Design review of the part built by this model. Coordinates are the model's own, in mm. A direction names the side the tool comes from. Give positions to 0.01 mm unless a question says otherwise; leave off trailing zeros. Order: outer loops, then holes, each group sorted by start corner. A loop starts at its lowest first (then second) coordinate and runs counter-clockwise, first axis right, second up. Notation, with made-up numbers: (-24.75, 83) -> (-17.75, 83) arc R29 ccw to (-17.75, 119) -> close; hole circle Ø1 at (61.25, -16). An arc over 180 degrees is marked (long way). One line per item, written item: value. Start each with the question number.
1) Tool access review of faces 1 (the face through (3, 4.3, -3)), 2 (the face through (149, 4, 10.3)), 3 (the face through (84, 0, 0)): name each direction out of +Z, -Z, +X, -X, +Y, -Y from which nothing blocks a thin tool from reaching the whole face with its end or side.
2) For pin 1 (3 mm diameter, centred on y = 2, z = 4.5, fed in from +X); pin 2 (1.8 mm diameter, centred on x = -6, z = 5.5, fed in from +Y); pin 3 (2 mm diameter, centred on x = 173.25, z = 5, fed in from +Y), all flat-tipped, find the tip position at first contact; note any pin that passes through.
3) The part is to be moulded in two halves that separate along Z. For faces 4 (the face through (-10.74, 6.18, -2.38)), 5 (the face through (84, 4, 17)), 6 (the face through (84, 8, 0)), say which applies: released by +Z, released by -Z, zero draft, split by the parting line, or undercut.
4) Consider section A-A (z = 0). State the section outline as (x, y) points.
5) Wall thickness on line 1 along Z through (x, y) = (125.75, 3.75); line 2 along Z through (x, y) = (153, 5); line 3 along X through (y, z) = (3, -5): over which ranges is each line inside the solid? List them lowest first. Write a range as from..to.
6) Consider section D-D (x = 173.25). State the section outline as (y, z) points, plus the area to 3 significant figures.
7) Consider section C-C (x = 139). State the section outline as (y, z) points, plus the area to 3 significant figures.
8) Consider section B-B (y = 2.5). State how many separate pieces and enclosed holes the cut face has, plus the area to 3 significant figures.
from build123d import *

# Parameters (mm, degrees)
ESTRUSIONE_ESTRUSIONE1_DEPTH  = 8
TAGLIO_ESTRUSIONE1_DEPTH      = 183.967210177
TAGLIO_ESTRUSIONE1_DEPTH_BACK = 183.967210177
SCHIZZO2_R                    = 3.5
SCHIZZO2_W                    = 41.6
SCHIZZO2_H                    = 20.6
SCHIZZO3_R                    = 11
TAGLIO_ESTRUSIONE2_DEPTH      = 3.7
SCHIZZO4_R                    = 1.1
TAGLIO_ESTRUSIONE3_DEPTH      = 3
SCHIZZO5_R                    = 1.75
TAGLIO_ESTRUSIONE4_DEPTH      = 183.967210177


with BuildPart() as part:
    # Schizzo1 → Estrusione-Estrusione1 (new body)
    with BuildSketch(Plane(origin=(0, 0, 0), x_dir=(1, 0, 0), z_dir=(0, 1, 0))):
        with BuildLine():
            Line((0, 17), (165, 17))
            ThreePointArc((165, 17), (182, 0), (165, -17))
            Line((165, -17), (0, -17))
            ThreePointArc((0, -17), (-17, 0), (0, 17))
        make_face()
    extrude(amount=ESTRUSIONE_ESTRUSIONE1_DEPTH)

    # Schizzo2 → Taglio-Estrusione1 (cut, two sides: drawn at the far end of the back side and taken through both)
    with BuildSketch(Plane.XZ.offset(-TAGLIO_ESTRUSIONE1_DEPTH_BACK)):
        with Locations(Location((0, 0, 0), (0, 0, 270))):
            Circle(SCHIZZO2_R)
        with Locations((149.5, 0)):
            Rectangle(SCHIZZO2_W, SCHIZZO2_H)
    extrude(amount=TAGLIO_ESTRUSIONE1_DEPTH + TAGLIO_ESTRUSIONE1_DEPTH_BACK, mode=Mode.SUBTRACT)

    # Schizzo3 → Taglio-Estrusione2 (cut)
    with BuildSketch(Plane(origin=(0, 8, 0), x_dir=(1, 0, 0), z_dir=(0, 1, 0))):
        with Locations(Location((0, 0, 0), (0, 0, 270))):
            Circle(SCHIZZO3_R)
    extrude(amount=-TAGLIO_ESTRUSIONE2_DEPTH, mode=Mode.SUBTRACT)

    # Schizzo4 → Taglio-Estrusione3 (cut)
    with BuildSketch(Plane(origin=(0, 4.3, 0), x_dir=(1, 0, 0), z_dir=(0, 1, 0))):
        with Locations(Location((-5.66, 5.66, 0), (0, 0, 270))):
            Circle(SCHIZZO4_R)
        with Locations(Location((5.66, 5.66, 0), (0, 0, 270))):
            Circle(SCHIZZO4_R)
        with Locations(Location((5.66, -5.66, 0), (0, 0, 270))):
            Circle(SCHIZZO4_R)
        with Locations(Location((-5.66, -5.66, 0), (0, 0, 270))):
            Circle(SCHIZZO4_R)
    extrude(amount=-TAGLIO_ESTRUSIONE3_DEPTH, mode=Mode.SUBTRACT)

    # Schizzo5 → Taglio-Estrusione4 (cut, through all)
    with BuildSketch(Plane(origin=(0, 8, 0), x_dir=(1, 0, 0), z_dir=(0, 1, 0))):
        with Locations(Location((125.75, 5, 0), (0, 0, 270))):
            Circle(SCHIZZO5_R)
        with Locations(Location((125.75, -5, 0), (0, 0, 270))):
            Circle(SCHIZZO5_R)
        with Locations(Location((173.25, -5, 0), (0, 0, 270))):
            Circle(SCHIZZO5_R)
        with Locations(Location((173.25, 5, 0), (0, 0, 270))):
            Circle(SCHIZZO5_R)
    extrude(amount=-TAGLIO_ESTRUSIONE4_DEPTH, mode=Mode.SUBTRACT)


solid = part.part
Checked values:
1. face 1: +Y
1. face 2: +Y, -Y
1. face 3: +Z, -Z, +X, -X, -Y
2. pin 1: stops at x = 181.73
2. pin 2: stops at y = 4.3
2. pin 3: passes through
3. face 4: undercut
3. face 5: released by +Z
3. face 6: zero draft
4. outline: (-17, 0) -> (-3.5, 0) -> (-3.5, 4.3) -> (-11, 4.3) -> (-11, 8) -> (-17, 8) -> close; (3.5, 0) -> (128.7, 0) -> (128.7, 8) -> (11, 8) -> (11, 4.3) -> (3.5, 4.3) -> close; (170.3, 0) -> (182, 0) -> (182, 8) -> (170.3, 8) -> close
5. line 1: z = -17..-6.75, -3.25..3.25, 6.75..17
5. line 2: z = -17..-10.3, 10.3..17
5. line 3: x = -16.25..-6.54, -4.78..4.78, 6.54..124, 127.5..128.7, 170.3..171.5, 175..181.25
6. outline: (0, -14.86) -> (8, -14.86) -> (8, -6.75) -> (0, -6.75) -> close; (0, -3.25) -> (8, -3.25) -> (8, 3.25) -> (0, 3.25) -> close; (0, 6.75) -> (8, 6.75) -> (8, 14.86) -> (0, 14.86) -> close
6. area: 182 mm^2
7. outline: (0, -17) -> (8, -17) -> (8, -10.3) -> (0, -10.3) -> close; (0, 10.3) -> (8, 10.3) -> (8, 17) -> (0, 17) -> close
7. area: 107 mm^2
8. separate pieces: 1
8. enclosed holes: 10
8. area: 5,570 mm^2
